Work out the finished part from the listing and answer in its coordinate system (mm). A direction names the side the tool comes from. Coordinates: 2 decimals unless noted, no trailing zeros. Write each loop counter-clockwise with the first axis right and the second up, starting at its lowest first coordinate (ties: lowest second). Pieces come first, ordered by that corner, then holes. Notation, with made-up numbers: (-23.5, 50.25) - (3.5, 50.25) arc R17 cw to (3.5, 59.25) - close; hole circle Ø1 at (55.25, 72). An arc over 180 degrees is marked (long way). Answer as a JSON object with one key per item and string values. Group by question number.
from build123d import *

# Parameters (mm, degrees)
SKETCH1_W                = 1.95
SKETCH1_H                = 9.75
SKETCH1_W_2              = 105
SKETCH1_H_2              = 4
BOSS_EXTRUDE1_DEPTH      = 12.45
SKETCH2_W                = 9.9
SKETCH2_H                = 8
SKETCH2_R                = 1.55
BOSS_EXTRUDE2_DEPTH      = 2
BOSS_EXTRUDE2_DEPTH_BACK = 1.95
BOSS_EXTRUDE3_REACH      = 8
SKETCH3_W                = 9.9
SKETCH3_H                = 24.9
SKETCH4_W                = 9.9
SKETCH4_H                = 8
SKETCH4_R                = 1.55
BOSS_EXTRUDE4_DEPTH      = 2
BOSS_EXTRUDE4_DEPTH_BACK = 1.95
BOSS_EXTRUDE5_REACH      = 8
SKETCH5_W                = 9.9
SKETCH5_H                = 24.9
SKETCH6_W                = 100.9
SKETCH6_H                = 2.05
CUT_EXTRUDE1_DEPTH       = 4.7
SKETCH7_W                = 100.9
SKETCH7_H                = 2.05
CUT_EXTRUDE2_DEPTH       = 4.7
FILLET1_R                = 2
FILLET2_R                = 3


with BuildPart() as part:
    # Sketch1 → Boss-Extrude1 (new body, symmetric)
    with BuildSketch(Plane(origin=(0, 0, 0), x_dir=(1, 0, 0), z_dir=(0, 1, 0))):
        Polygon((-52.5, 63.25), (-52.5, 2), (-48.5, 2), (-48.5, 63.25), (-50.45, 63.25), align=None)
        with Locations((-49.475, 68.125)):
            Rectangle(SKETCH1_W, SKETCH1_H)
        Rectangle(SKETCH1_W_2, SKETCH1_H_2)
        Polygon((48.5, 63.25), (48.5, 2), (52.5, 2), (52.5, 63.25), (50.45, 63.25), align=None)
        with Locations((49.475, 68.125)):
            Rectangle(SKETCH1_W, SKETCH1_H)
    extrude(amount=BOSS_EXTRUDE1_DEPTH, both=True)

    # Sketch2 → Boss-Extrude2 (add, two sides)
    with BuildSketch(Plane.ZY.offset(-48.5)) as boss_extrude2_sk:
        with Locations((-16, -16.45)):
            Rectangle(SKETCH2_W, SKETCH2_H)
        with Locations((-16, -16.5)):
            Circle(SKETCH2_R, mode=Mode.SUBTRACT)
        with Locations((-44, -16.45)):
            Rectangle(SKETCH2_W, SKETCH2_H)
        with Locations((-44, -16.5)):
            Circle(SKETCH2_R, mode=Mode.SUBTRACT)
        with Locations((-16, 16.45)):
            Rectangle(SKETCH2_W, SKETCH2_H)
        with Locations((-16, 16.5)):
            Circle(SKETCH2_R, mode=Mode.SUBTRACT)
        with Locations((-44, 16.45)):
            Rectangle(SKETCH2_W, SKETCH2_H)
        with Locations((-44, 16.5)):
            Circle(SKETCH2_R, mode=Mode.SUBTRACT)
    extrude(amount=BOSS_EXTRUDE2_DEPTH)
    extrude(boss_extrude2_sk.sketch, amount=-BOSS_EXTRUDE2_DEPTH_BACK)

    # Sketch3 → Boss-Extrude3 (add, up to next)
    with BuildSketch(Plane.ZY.offset(-46.5), mode=Mode.PRIVATE) as boss_extrude3_sk1:
        with Locations((-44, 0)):
            Rectangle(SKETCH3_W, SKETCH3_H)
    boss_extrude3_tool1 = extrude(boss_extrude3_sk1.sketch, amount=-BOSS_EXTRUDE3_REACH, mode=Mode.PRIVATE) - part.part
    add(boss_extrude3_tool1.solids().sort_by_distance((46.5, 0, -44))[0])
    # Sketch3 → Boss-Extrude3 (add, up to next)
    with BuildSketch(Plane.ZY.offset(-46.5), mode=Mode.PRIVATE) as boss_extrude3_sk2:
        with Locations((-16, 0)):
            Rectangle(SKETCH3_W, SKETCH3_H)
    boss_extrude3_tool2 = extrude(boss_extrude3_sk2.sketch, amount=-BOSS_EXTRUDE3_REACH, mode=Mode.PRIVATE) - part.part
    add(boss_extrude3_tool2.solids().sort_by_distance((46.5, 0, -16))[0])

    # Sketch4 → Boss-Extrude4 (add, two sides)
    with BuildSketch(Plane(origin=(-48.5, 0, 0), x_dir=(0, 0, -1), z_dir=(1, 0, 0))) as boss_extrude4_sk:
        with Locations((16, 16.45)):
            Rectangle(SKETCH4_W, SKETCH4_H)
        with Locations((16, 16.5)):
            Circle(SKETCH4_R, mode=Mode.SUBTRACT)
        with Locations((44, 16.45)):
            Rectangle(SKETCH4_W, SKETCH4_H)
        with Locations((44, 16.5)):
            Circle(SKETCH4_R, mode=Mode.SUBTRACT)
        with Locations((44, -16.45)):
            Rectangle(SKETCH4_W, SKETCH4_H)
        with Locations((44, -16.5)):
            Circle(SKETCH4_R, mode=Mode.SUBTRACT)
        with Locations((16, -16.45)):
            Rectangle(SKETCH4_W, SKETCH4_H)
        with Locations((16, -16.5)):
            Circle(SKETCH4_R, mode=Mode.SUBTRACT)
    extrude(amount=BOSS_EXTRUDE4_DEPTH)
    extrude(boss_extrude4_sk.sketch, amount=-BOSS_EXTRUDE4_DEPTH_BACK)

    # Sketch5 → Boss-Extrude5 (add, up to next)
    with BuildSketch(Plane(origin=(-46.5, 0, 0), x_dir=(0, 0, -1), z_dir=(1, 0, 0)), mode=Mode.PRIVATE) as boss_extrude5_sk1:
        with Locations((16, 0)):
            Rectangle(SKETCH5_W, SKETCH5_H)
    boss_extrude5_tool1 = extrude(boss_extrude5_sk1.sketch, amount=-BOSS_EXTRUDE5_REACH, mode=Mode.PRIVATE) - part.part
    add(boss_extrude5_tool1.solids().sort_by_distance((-46.5, 0, -16))[0])
    # Sketch5 → Boss-Extrude5 (add, up to next)
    with BuildSketch(Plane(origin=(-46.5, 0, 0), x_dir=(0, 0, -1), z_dir=(1, 0, 0)), mode=Mode.PRIVATE) as boss_extrude5_sk2:
        with Locations((44, 0)):
            Rectangle(SKETCH5_W, SKETCH5_H)
    boss_extrude5_tool2 = extrude(boss_extrude5_sk2.sketch, amount=-BOSS_EXTRUDE5_REACH, mode=Mode.PRIVATE) - part.part
    add(boss_extrude5_tool2.solids().sort_by_distance((-46.5, 0, -44))[0])

    # Sketch6 → Cut-Extrude1 (cut)
    with BuildSketch(Plane.XZ.offset(12.45)):
        with Locations((0, 0.975)):
            Rectangle(SKETCH6_W, SKETCH6_H)
        Polygon((50.45, 2), (50.45, -0.05), (50.45, -63.25), (52.5, -63.25), (52.5, 2), align=None)
        Polygon((-52.5, -63.25), (-50.45, -63.25), (-50.45, -0.05), (-50.45, 2), (-52.5, 2), align=None)
    extrude(amount=-CUT_EXTRUDE1_DEPTH, mode=Mode.SUBTRACT)

    # Sketch7 → Cut-Extrude2 (cut)
    with BuildSketch(Plane(origin=(0, 12.45, 0), x_dir=(1, 0, 0), z_dir=(0, 1, 0))):
        Polygon((-50.45, 48.95), (-50.45, 63.25), (-52.5, 63.25), (-52.5, -2), (-50.45, -2), (-50.45, 0.05), (-50.45, 11.05), (-50.45, 20.95), (-50.45, 39.05), align=None)
        with Locations((0, -0.975)):
            Rectangle(SKETCH7_W, SKETCH7_H)
        Polygon((50.45, 0.05), (50.45, -2), (52.5, -2), (52.5, 63.25), (50.45, 63.25), (50.45, 48.95), (50.45, 39.05), (50.45, 20.95), (50.45, 11.05), align=None)
    extrude(amount=-CUT_EXTRUDE2_DEPTH, mode=Mode.SUBTRACT)

    # Fillet1
    fillet1_edges = [part.edges().sort_by_distance(p)[0] for p in [
        (-49.475, 12.45, -11.05),
        (-49.475, 12.45, -20.95),
        (-49.475, 12.45, -39.05),
        (-49.475, 12.45, -48.95),
        (-49.475, -12.45, -39.05),
        (-49.475, -12.45, -48.95),
        (-49.475, -12.45, -11.05),
        (-49.475, -12.45, -20.95),
        (49.475, -12.45, -20.95),
        (49.475, -12.45, -11.05),
        (49.475, -12.45, -48.95),
        (49.475, -12.45, -39.05),
        (49.475, 12.45, -11.05),
        (49.475, 12.45, -20.95),
        (49.475, 12.45, -48.95),
        (49.475, 12.45, -39.05),
    ]]
    fillet(fillet1_edges, radius=FILLET1_R)

    # Fillet2
    fillet2_edges = [part.edges().sort_by_distance(p)[0] for p in [
        (-48.5, 0, -2),
        (48.5, 0, -2),
    ]]
    fillet(fillet2_edges, radius=FILLET2_R)


solid = part.part
Q1. For a pull along Z with two mould halves and no side action, classify faces 4 (the face through (-48, 20.45, -16)), 5 (the face through (-48.5, 0, -30)), 6 (the face through (-48, 0, -48.95)), 7 (the face through (-47.6, 0.17, -2.86)) as +Z half, -Z half, draft (parallel to the pull), parting line (faces both ways), or undercut.
Q2. Consider L1, parallel to Y at x = -47.25, z = -44; L2, parallel to X at y = -10, z = -56.5; L3, parallel to Z at x = 48, y = 16. Determine where each line is inside the solid, lowest interval first. Write a range as from..to.
Q3. Flat-ended cylindrical pins translate along their axes: pin 1 Ø1.9 at (y, z) = (-16.5, -16) entering from +X; pin 2 Ø12.5 at (x, y) = (11, 5.5) entering from -Z; pin 3 Ø4.5 at (x, z) = (-25, -2.5) entering from +Y; pin 4 Ø1.5 at (y, z) = (-12, -56) entering from +X. Find the tip coordinate at first contact, or state that the pin passes through.
Q4. Section C-C on x = -20.5 is taken. Determine the outline of the cut face in (y, z), plus the area to 3 significant figures.
Q5. Section A-A on z = -44 is taken. Count the separate pieces of the cut face and the enclosed holes in it, plus the area to 3 significant figures.
Q6. A tool of negligible diameter and unlimited length cuts with its end or side. For faces 1 (the face through (-4, -12.45, -1.6)), 2 (the face through (49, 20.45, -44)), 3 (the face through (46.5, 0, -16)), from which of +Z, -Z, +X, -X, +Y, -Y can it reach the whole face along a straight path? Write none if from no direction.
Numbers:
{
 "1": {"face 4": "draft", "face 5": "undercut", "face 6": "-Z half", "face 7": "undercut"},
 "2": {"L1": "y = -20.45..-18.05, -14.95..14.95, 18.05..20.45", "L2": "x = -50.45..-48.5, 48.5..50.45", "L3": "z = -48.95..-45.47, -42.53..-39.05, -20.95..-17.47, -14.53..-11.05"},
 "3": {"pin 1": "passes through", "pin 2": "stops at z = -2", "pin 3": "stops at y = 12.45", "pin 4": "stops at x = 50.45"},
 "4": {"outline": "(-12.45, -2) - (12.45, -2) - (12.45, -0.05) - (7.75, -0.05) - (7.75, 2) - (-7.75, 2) - (-7.75, -0.05) - (-12.45, -0.05) - close", "area": "80.3 mm²"},
 "5": {"separate pieces": "6", "enclosed holes": "0", "area": "338 mm²"},
 "6": {"face 1": "+Z, +X, -X, -Y", "face 2": "+Z, -Z, +X, -X, +Y", "face 3": "-Z, +Y, -Y"}
}
